Source: CAD feature listing. Evaluate the final solid. Frame: model axes, mm. A direction names the side the tool comes from. Coordinates: 2 decimals unless noted, no trailing zeros. Order: outer loops, then holes, each group sorted by start corner. A loop starts at its lowest first (then second) coordinate and runs counter-clockwise, first axis right, second up.
```python
from build123d import *

# Parameters (mm, degrees)
SKETCH4_OUTSIDE_W           = 16.898
SKETCH4_OUTSIDE_H           = 16.898
SKETCH4_OUTSIDE_W_2         = 32
SKETCH4_OUTSIDE_H_2         = 9
CUT_EXTRUDE1_DEPTH          = 21
F_1_4_28_TAPPED_HOLE2_D     = 5.4102
F_1_4_28_TAPPED_HOLE2_DEPTH = 10
M3_TAPPED_HOLE1_D           = 2.5


with BuildPart() as part:
    # Sketch1 → Revolve1 (revolve)
    with BuildSketch(Plane.XY):
        Polygon((-1.315886695, -5.259279322), (-4.815886695, -5.259279322), (-4.815886695, -4.759279322), (-5.815886695, -5.259279322), (-6.315886695, -5.259279322), (-6.315886695, -4.759279322), (-7.315886695, -5.259279322), (-7.815886695, -5.259279322), (-7.815886695, -4.759279322), (-8.815886695, -5.259279322), (-9.315886695, -5.259279322), (-9.315886695, -5.759279322), (0.684113305, -5.759279322), (0.684113305, -7.759279322), (10.684113305, -7.759279322), (10.684113305, -2.759279322), (-1.315886695, -2.759279322), align=None)
    revolve(axis=Axis((2.271553965, -7.759279322, 0), (-1, 0, 0)))

    # Sketch4 outside → Cut-Extrude1 (cut, through all)
    with BuildSketch(Plane(origin=(10.684113305, 0, 0), x_dir=(0, 0, -1), z_dir=(1, 0, 0))):
        with Locations((0, -7.759)):
            Rectangle(SKETCH4_OUTSIDE_W, SKETCH4_OUTSIDE_H)
        with Locations((0, -7.759279322)):
            Rectangle(SKETCH4_OUTSIDE_W_2, SKETCH4_OUTSIDE_H_2, mode=Mode.SUBTRACT)
    extrude(amount=-CUT_EXTRUDE1_DEPTH, mode=Mode.SUBTRACT)

    # 1/4-28 Tapped Hole2
    with Locations(Plane(origin=(10.684113305, 0, 0), x_dir=(0, 0, -1), z_dir=(1, 0, 0))):
        with Locations((0, -7.759279322)):
            Hole(F_1_4_28_TAPPED_HOLE2_D / 2, depth=F_1_4_28_TAPPED_HOLE2_DEPTH)

    # M3 Tapped Hole1 (through all)
    with Locations(Plane(origin=(0, -3.259279322, 0), x_dir=(1, 0, 0), z_dir=(0, 1, 0))):
        with Locations((3.162442737, 0)):
            Hole(M3_TAPPED_HOLE1_D / 2)


solid = part.part
```
Q1. Section query A-A on x = 4. Output: boundary loops of the cut face in (y, z).
Solutions:
outline: (-12.26, -2.18) arc R5 ccw to (-3.26, -2.18) - (-3.26, -0.93) - (-5.22, -0.93) arc R2.71 cw to (-10.3, -0.93) - (-12.26, -0.93) - close; (-12.26, 0.93) - (-10.3, 0.93) arc R2.71 cw to (-5.22, 0.93) - (-3.26, 0.93) - (-3.26, 2.18) arc R5 ccw to (-12.26, 2.18) - close
Q2. Material intervals for line 1 along Y through (x, z) = (-4.25, 0); line 2 along X through (y, z) = (-11, -3.75); line 3 along Y through (x, z) = (0, -1), sorted ascending.
Solutions:
line 1: y = -10.26 to -9.76, -5.76 to -5.26
line 2: x = -1.32 to 10.68
line 3: y = -12.26 to -9.49, -6.03 to -3.26
Q3. Section query B-B on z = 0. Give the number of separate pieces and of enclosed holes in the cut face, plus the area to 3 significant figures.
Solutions:
separate pieces: 4
enclosed holes: 0
area: 46.4 mm2
Q4. Section query C-C on x = 1.25. Output: boundary loops of the cut face in (y, z).
Solutions:
outline: (-12.26, -2.18) arc R5 ccw to (-3.26, -2.18) - (-3.26, 2.18) arc R5 ccw to (-12.26, 2.18) - close; hole circle Ø5.41 at (-7.76, 0)
Q5. Section query D-D on y = -11. Output: boundary loops of the cut face in (x, z).
Solutions:
outline: (-1.32, -3.81) - (10.68, -3.81) - (10.68, 3.81) - (-1.32, 3.81) - close; hole circle Ø2.5 at (3.16, 0)
Q6. Pull-direction query (X, two-part tool) for faces 1 (the cylindrical face through (1.97, -4.32, -0.38)), 2 (the flat face through (0.684, -9, -2)), 3 (the flat face through (5, -3.259, 0)); classes: pulls with the +X half, pulls with the -X half, needs draft (parallel to the pull), parting line crosses it, or undercut.
Solutions:
face 1: undercut
face 2: pulls with the +X half
face 3: needs draft
Q7. Pin query (flat end, axial travel): P1, Ø1.5, axis at y = -11, z = -2, coming from the -X side; P2, Ø1.5, axis at y = -9.5, z = -0.5, coming from the +X side; P3, Ø1.5, axis at y = -8.5, z = -0.5, coming from the +X side. Return the tip coordinate at first contact, or that it passes through.
Solutions:
P1: stops at x = -1.32
P2: stops at x = 0.68
P3: passes through
Q8. Set-up query: faces 4 (the cylindrical face through (-4.246, -9.757, -0.088)), 5 (the cylindrical face through (4.6, -7.7, -5)), 6 (the flat face through (-4.816, -6, -2)), 7 (the cylindrical face through (-9.07, -8.3, 2.44)), 8 (the cylindrical face through (5.614, -8.795, 2.499)). Return all of +Z, -Z, +X, -X, +Y, -Y with unobstructed straight access to the full face (end or side cutting, diameter ignored); none if empty.
Solutions:
face 4: +X, -X
face 5: -Z, +X, -X
face 6: none
face 7: -X
face 8: +X
